Autodesk Inventor part; units mm, degrees
ref_plane "YZ Plane" through (0, 0, 0) normal (1, 0, 0) x (0, 1, 0)
ref_plane "XZ Plane" through (0, 0, 0) normal (0, 1, 0) x (-1, 0, 0)
ref_plane "XY Plane" through (0, 0, 0) normal (0, 0, 1) x (1, 0, 0)
sketch "Skizze1" plane through (0, 0, 0) normal (0, 1, 0) x (-1, 0, 0)
  line L0 (6.725, 3.8827) -> (6.725, -3.8827)
  line L1 (6.725, -3.8827) -> (0, -7.7654)
  line L2 (0, -7.7654) -> (-6.725, -3.8827)
  line L3 (-6.725, -3.8827) -> (-6.725, 3.8827)
  line L4 (-6.725, 3.8827) -> (0, 7.7654)
  line L5 (0, 7.7654) -> (6.725, 3.8827)
  line L6 (-8, -8) -> (8, -8)
  line L7 (8, -8) -> (8, 8)
  line L8 (8, 8) -> (-8, 8)
  line L9 (-8, 8) -> (-8, -8)
  line L10 (-8, -8) -> (8, 8) construction
  line L11 (8, -8) -> (-8, 8) construction
  point P0 (0, 0)
  point P1 (0, 0)
  point P2 (-0.3096, 7.5)
  point P3 (-0.3096, -7.5)
  point P4 (0.3096, -7.5)
  point P5 (0.3096, 7.5)
  dimension "d0" = 16
  dimension "d1" = 16
  dimension "d2" = 13.45
extrude "Extrusion1" add sketch "Skizze1" along normal blind 3
fillet "Rundung1" radius 2 6 edges at (-6.725, 1.5, -3.8827) (-6.725, 1.5, 3.8827) (0, 1.5, 7.7654) (6.725, 1.5, 3.8827) (6.725, 1.5, -3.8827) (0, 1.5, -7.7654)
sketch "Skizze2" plane through (0, 3, 0) normal (0, 1, 0) x (1, 0, 0)
  line L0 (-8, 8) -> (-8, -8)
  line L1 (-8, -8) -> (8, -8)
  line L2 (8, -8) -> (8, 8)
  line L3 (8, 8) -> (-8, 8)
  line L4 (-5.725, 4.46) -> (-1, 7.188)
  arc A0 (1, 7.188) -> (-1, 7.188) centre (0, 5.456) ccw
  line L5 (1, 7.188) -> (5.725, 4.46)
  arc A1 (6.725, 2.728) -> (5.725, 4.46) centre (4.725, 2.728) ccw
  line L6 (6.725, 2.728) -> (6.725, -2.728)
  arc A2 (5.725, -4.46) -> (6.725, -2.728) centre (4.725, -2.728) ccw
  line L7 (5.725, -4.46) -> (1, -7.188)
  arc A3 (-1, -7.188) -> (1, -7.188) centre (0, -5.456) ccw
  line L8 (-1, -7.188) -> (-5.725, -4.46)
  arc A4 (-6.725, -2.728) -> (-5.725, -4.46) centre (-4.725, -2.728) ccw
  line L9 (-6.725, -2.728) -> (-6.725, 2.728)
  arc A5 (-5.725, 4.46) -> (-6.725, 2.728) centre (-4.725, 2.728) ccw
  line L10 (0, -6.8416) -> (-5.925, -3.4208)
  line L11 (-5.925, -3.4208) -> (-5.925, 3.4208)
  line L12 (-5.925, 3.4208) -> (0, 6.8416)
  line L13 (0, 6.8416) -> (5.925, 3.4208)
  line L14 (5.925, 3.4208) -> (5.925, -3.4208)
  line L15 (5.925, -3.4208) -> (0, -6.8416)
  point P0 (0, 0)
  point P1 (0, 0)
  point P2 (8, 5.7735)
  point P3 (8, -5.7735)
  point P4 (-8, -5.7735)
  point P5 (-8, 5.7735)
  point P6 (4.1436, -8)
  point P7 (-4.1436, -8)
  point P8 (4.1436, 8)
  point P9 (-4.1436, 8)
  dimension "d6" = 11.85
extrude "Extrusion2" add sketch "Skizze2" along normal blind 13 contours L3 L2 L1 L0 | L4 A0 L5 A1 L6 A2 L7 A3 L8 A4 L9 A5
fillet "Rundung2" radius 1 16 edges at (0, 9.5, 6.8416) (-5.925, 9.5, 3.4208) (-5.925, 9.5, -3.4208) (0, 9.5, -6.8416) (5.925, 9.5, -3.4208) (5.925, 9.5, 3.4208) (8, 8, -8) (-8, 8, -8) (-8, 8, 8) (8, 8, 8) (-2.9625, 16, -5.1312) (-5.925, 16, 0) (-2.9625, 16, 5.1312) (2.9625, 16, 5.1312) (5.925, 16, 0) (2.9625, 16, -5.1312)
ref_plane "Arbeitsebene1" through (0, 0, -8) normal (-1, 0, 0) x (0, 0, 1)
ref_plane "Arbeitsebene2" through (-8, 0, 0) normal (0, 0, 1) x (1, 0, 0)
sketch "Skizze3" plane through (0, 16, 0) normal (0, 1, 0) x (1, 0, 0)
  arc A0 (7, -8) -> (8, -7) centre (7, -7) ccw
  line L0 (8, -7) -> (8, 7)
  arc A1 (8, 7) -> (7, 8) centre (7, 7) ccw
  line L1 (7, 8) -> (-7, 8)
  arc A2 (-7, 8) -> (-8, 7) centre (-7, 7) ccw
  line L2 (-8, 7) -> (-8, -7)
  arc A3 (-8, -7) -> (-7, -8) centre (-7, -7) ccw
  line L3 (-7, -8) -> (7, -8)
  arc A4 (-1, -7.419) -> (1, -7.419) centre (0, -5.6869) ccw
  line L4 (-5.925, -4.5755) -> (-1, -7.419)
  arc A5 (-6.925, -2.8435) -> (-5.925, -4.5755) centre (-4.925, -2.8435) ccw
  line L5 (-6.925, 2.8435) -> (-6.925, -2.8435)
  arc A6 (-5.925, 4.5755) -> (-6.925, 2.8435) centre (-4.925, 2.8435) ccw
  line L6 (-1, 7.419) -> (-5.925, 4.5755)
  arc A7 (1, 7.419) -> (-1, 7.419) centre (0, 5.6869) ccw
  line L7 (5.925, 4.5755) -> (1, 7.419)
  arc A8 (6.925, 2.8435) -> (5.925, 4.5755) centre (4.925, 2.8435) ccw
  line L8 (6.925, -2.8435) -> (6.925, 2.8435)
  arc A9 (5.925, -4.5755) -> (6.925, -2.8435) centre (4.925, -2.8435) ccw
  line L9 (1, -7.419) -> (5.925, -4.5755)
  line L10 (-8, -5.6869) -> (8, -5.6869)
  line L11 (8, -5.6869) -> (8, -13.6869)
  line L12 (6, -15.6869) -> (-6, -15.6869)
  line L13 (-8, -13.6869) -> (-8, -5.6869)
  circle A10 centre (-4.925, -12.0977) radius 1.4
  circle A11 centre (2.836, -12.0977) radius 1.4
  arc A12 (-8, -13.6869) -> (-6, -15.6869) centre (-6, -13.6869) ccw
  arc A13 (6, -15.6869) -> (8, -13.6869) centre (6, -13.6869) ccw
  point P0 (0, 0)
  point P1 (8, -15.6869)
  point P2 (8, -7)
  dimension "d10" = 10
  dimension "d11" = 2.8
  dimension "d12" = 2.8
  dimension "d13" = 2
extrude "Extrusion3" add sketch "Skizze3" against normal blind 3 contours A0 L11 A13 L12 A12 L13 A3 L3
sketch "Skizze4" plane through (0, 0, 0) normal (0, -1, 0) x (1, 0, 0)
  line L0 (12.8, 30) -> (12.8, 10)
  line L1 (12.8, 30) -> (6.8, 30)
  line L2 (6.8, 10) -> (6.8, 30)
  line L3 (12.8, 10) -> (6.8, 10)
  line L4 (6.7, 30.1) -> (12.9, 30.1)
  line L5 (12.9, 30.1) -> (12.9, 9.9)
  line L6 (12.9, 9.9) -> (6.7, 9.9)
  line L7 (6.7, 9.9) -> (6.7, 30.1)
  point P0 (0, 0)
  dimension "d16" = 0.1
extrude "Extrusion4" cut sketch "Skizze4" against normal through all contours L0 L3 L2 L1 | L4 L5 L6 L7
sketch "Skizze5" plane through (0, 0, 0) normal (0, -1, 0) x (1, 0, 0)
  line L0 (-4.75, -4.75) -> (4.75, -4.75)
  line L1 (4.75, -4.75) -> (4.75, 4.75)
  line L2 (4.75, 4.75) -> (-4.75, 4.75)
  line L3 (-4.75, 4.75) -> (-4.75, -4.75)
  line L4 (-4.75, -4.75) -> (4.75, 4.75) construction
  line L5 (4.75, -4.75) -> (-4.75, 4.75) construction
  point P0 (0, 0)
  dimension "d19" = 9.5
  dimension "d20" = 9.5
properties part number "30_Laser_to_M12Adapter"
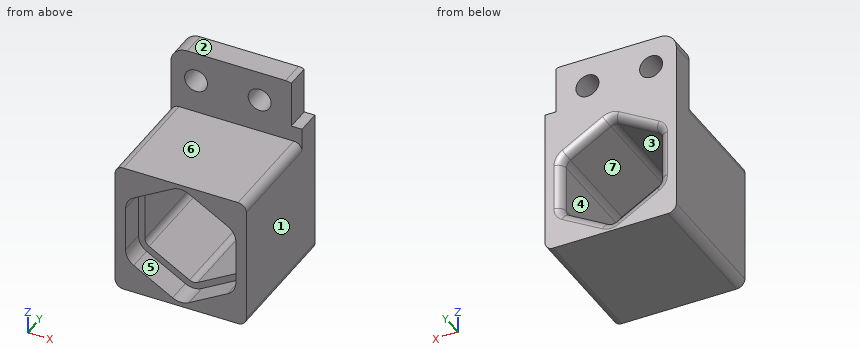
Could you check a few things on this model? Use its own coordinates, in mm. Face numbers are marked on the shaded views. A direction names the side the tool comes from. Give positions to 0.01 mm unless a question says otherwise; leave off trailing zeros. Order: outer loops, then holes, each group sorted by start corner. A loop starts at its lowest first (then second) coordinate and runs counter-clockwise, first axis right, second up. Notation, with made-up numbers: (-11.5, 15) -> (10.5, 15) arc R21 ccw to (10.5, 37) -> close; hole circle Ø3 at (1, -9). An arc over 180 degrees is marked (long way). Return JSON: item names as keys, results as strings.
1. For pin 1 Ø3.5 at (x, z) = (-4.92, 12.1) entering from -Y; pin 2 Ø1.5 at (y, z) = (14.5, 12.5) entering from +X; pin 3 Ø3 at (x, y) = (2, 10) entering from +Z, each with a flat end and sliding along its axis, tell me the tip position at first contact or that it passes through.
Answer list:
{"pin 1": "stops at y = 13", "pin 2": "stops at x = 6.7", "pin 3": "stops at z = 8"}
2. Thinking about a two-plate mould opening in Z: for the marked faces 1, 2, 3 and 4, which applies, pulls with the +Z half, pulls with the -Z half, needs draft (parallel to the pull), parting line crosses it, or undercut?
Answer list:
{"face 1": "needs draft", "face 2": "pulls with the +Z half", "face 3": "undercut", "face 4": "undercut"}
3. Imagine slicing it at B-B on z = 2. List the corners of the cut face in (x, y) for me (3 decimals), then the cut area to 3 significant figures.
Answer list:
{"outline": "(-8, 0) -> (-6.725, 0) -> (-6.725, 3) -> (-5.925, 3) -> (-5.925, 15) arc R1 ccw to (-6.925, 16) -> (-8, 16) -> close; (5.925, 3) -> (6.725, 3) -> (6.725, 0) -> (8, 0) -> (8, 16) -> (6.925, 16) arc R1 ccw to (5.925, 15) -> close", "area": "61.2 mm2"}
4. On a 3-axis mill with a long thin cutter (end or side, diameter ignored), from which of +Z, -Z, +X, -X, +Y, -Y can I reach the whole of each face in a straight line? I mean the marked faces 5, 6 and 7. Say none if no direction works.
Answer list:
{"face 5": "-Y", "face 6": "+Z, +X, -X, -Y", "face 7": "+Y, -Y"}
5. Imagine slicing it at C-C on y = 13.5. List the corners of the cut face in (x, z) for me (3 decimals).
Answer list:
{"outline": "(-8, -7) arc R1 ccw to (-7, -8) -> (7, -8) arc R1 ccw to (8, -7) -> (8, 9.9) -> (6.7, 9.9) -> (6.7, 15.56) arc R2 ccw to (6, 15.687) -> (-6, 15.687) arc R2 ccw to (-8, 13.687) -> close; hole circle Ø2.8 at (-4.925, 12.098); hole (-5.925, -2.843) arc R1 ccw to (-5.425, -3.709) -> (-0.5, -6.553) arc R1 ccw to (0.5, -6.553) -> (5.425, -3.709) arc R1 ccw to (5.925, -2.843) -> (5.925, 2.843) arc R1 ccw to (5.425, 3.709) -> (0.5, 6.553) arc R1 ccw to (-0.5, 6.553) -> (-5.425, 3.709) arc R1 ccw to (-5.925, 2.843) -> close; hole circle Ø2.8 at (2.836, 12.098)"}
6. Imagine slicing it at A-A on y = 6. List the corners of the cut face in (x, z) for me (3 decimals), then the cut area to 3 significant figures.
Answer list:
{"outline": "(-8, -7) arc R1 ccw to (-7, -8) -> (7, -8) arc R1 ccw to (8, -7) -> (8, 7) arc R1 ccw to (7, 8) -> (-7, 8) arc R1 ccw to (-8, 7) -> close; hole (-5.925, -2.843) arc R1 ccw to (-5.425, -3.709) -> (-0.5, -6.553) arc R1 ccw to (0.5, -6.553) -> (5.425, -3.709) arc R1 ccw to (5.925, -2.843) -> (5.925, 2.843) arc R1 ccw to (5.425, 3.709) -> (0.5, 6.553) arc R1 ccw to (-0.5, 6.553) -> (-5.425, 3.709) arc R1 ccw to (-5.925, 2.843) -> close", "area": "134 mm2"}
7. Imagine slicing it at D-D on x = -4. Give the number of separate pieces and of enclosed holes in the cut face, then the cut area to 3 significant figures.
Answer list:
{"separate pieces": "3", "enclosed holes": "0", "area": "122 mm2"}
8. I need wall thicknesses on line 1 (Z direction, x = -0.5, y = 15); line 2 (Z direction, x = -0.5, y = 11.25); line 3 (X direction, y = 15, z = -1.5) (3 decimals). Which ranges of each line are inside material? Lowest first, please. Write a range as from..to.
Answer list:
{"line 1": "z = -8..-6.55, 6.55..15.69", "line 2": "z = -8..-6.55, 6.55..8", "line 3": "x = -8..-5.925, 5.925..8"}
